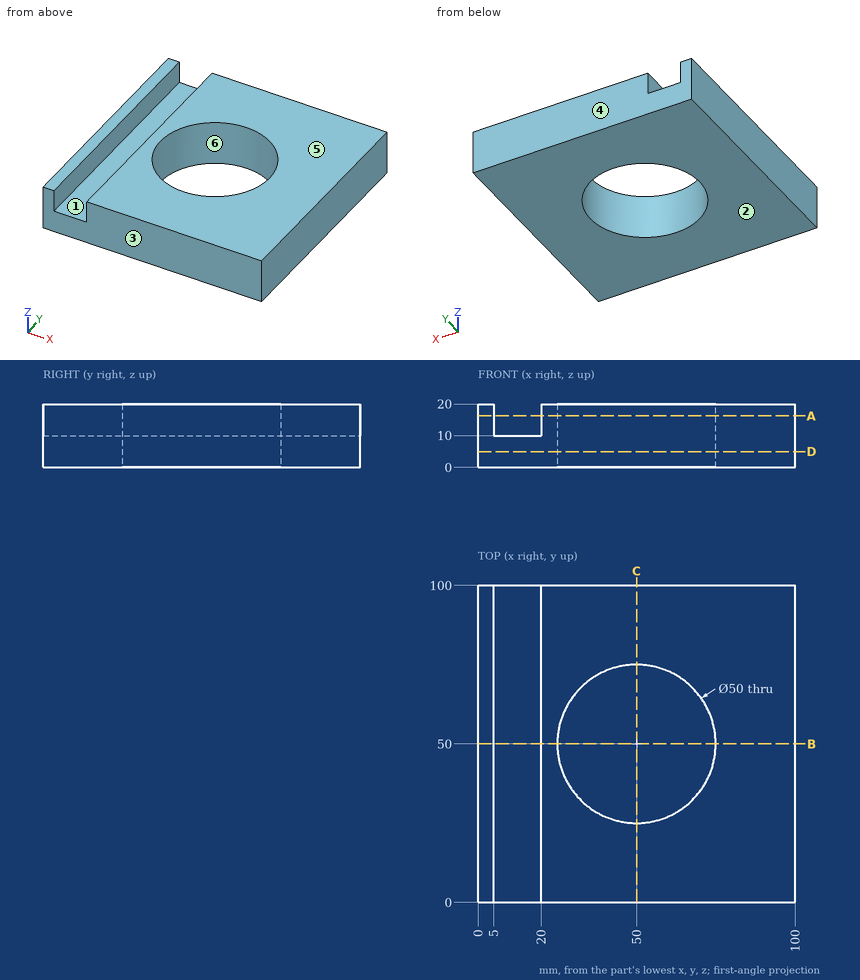
Geometry check sheet. Reference: drawing and pictorial views, mm from the part's lowest x, y, z. A direction names the side the tool comes from. Give positions to 0.01 mm unless a question says otherwise; leave off trailing zeros. Write each loop counter-clockwise with the first axis right and the second up, starting at its lowest first coordinate (ties: lowest second). Pieces come first, ordered by that corner, then holes. Notation, with made-up numbers: (-33, 3) - (21, 3) arc R25 ccw to (21, 35) - close; hole circle Ø6 at (77.25, -22.75). An arc over 180 degrees is marked (long way). Use a Markdown table: item, result.
Q1. Section check A-A, the plane z = 16.25. Enter the section's corners in (x, y), then the cut area to 3 significant figures.
Computed:
| item | result |
|---|---|
| outline | (0, 0) - (5, 0) - (5, 100) - (0, 100) - close; (20, 0) - (100, 0) - (100, 100) - (20, 100) - close; hole circle Ø50 at (50, 50) |
| area | 6,540 mm² |
Q2. Section check C-C, the plane x = 50. Enter the section's corners in (y, z), then the cut area to 3 significant figures.
Computed:
| item | result |
|---|---|
| outline | (0, 0) - (25, 0) - (25, 20) - (0, 20) - close; (75, 0) - (100, 0) - (100, 20) - (75, 20) - close |
| area | 1,000 mm² |
Q3. Section check B-B, the plane y = 50. Enter the section's corners in (x, z), then the cut area to 3 significant figures.
Computed:
| item | result |
|---|---|
| outline | (0, 0) - (25, 0) - (25, 20) - (20, 20) - (20, 10) - (5, 10) - (5, 20) - (0, 20) - close; (75, 0) - (100, 0) - (100, 20) - (75, 20) - close |
| area | 850 mm² |
Q4. Set-up check for the marked faces 1 and 2: record each of +Z, -Z, +X, -X, +Y, -Y from which the full face is reachable in a straight line by a thin tool's end or side.
Computed:
| item | result |
|---|---|
| face 1 | +Z, +Y, -Y |
| face 2 | -Z, +X, -X, +Y, -Y |
Q5. Draft check along Y on the marked faces 3, 4, 5 and 6. Enter one of: pulls with the +Y half, pulls with the -Y half, needs draft (parallel to the pull), parting line crosses it, or undercut.
Computed:
| item | result |
|---|---|
| face 3 | pulls with the -Y half |
| face 4 | pulls with the +Y half |
| face 5 | needs draft |
| face 6 | undercut |
Q6. Thickness scan on L1, parallel to X at y = 37, z = 11.5; L2, parallel to X at y = 28, z = 11; L3, parallel to Y at x = 50, z = 10.5. Record the ranges inside material, lowest first. Write a range as [from, to].
Computed:
| item | result |
|---|---|
| L1 | x = [0, 5], [20, 28.65], [71.35, 100] |
| L2 | x = [0, 5], [20, 38.13], [61.87, 100] |
| L3 | y = [0, 25], [75, 100] |
Q7. Section check D-D, the plane z = 5. Enter the section's corners in (x, y).
Computed:
| item | result |
|---|---|
| outline | (0, 0) - (100, 0) - (100, 100) - (0, 100) - close; hole circle Ø50 at (50, 50) |
